Check sheet for the modelled part. Datum: model origin and axes. Units: mm. A direction names the side the tool comes from. Round coordinates to 2 decimals unless told otherwise and drop trailing zeros. Write each loop counter-clockwise with the first axis right and the second up, starting at its lowest first coordinate (ties: lowest second). Pieces come first, ordered by that corner, then holes. Notation, with made-up numbers: (-37, 14.5) -> (2, 14.5) arc R23 ccw to (2, 31.5) -> close; hole circle Ø6 at (-33.75, 49). An arc over 180 degrees is marked (long way). Use one line per item in the form item = value. Start each with the question number.
```python
from build123d import *

# Parameters (mm, degrees)
F0_W     = 60
F0_H     = 20
F2_R     = 5
F3_DEPTH = 20
F4_R     = 5


with BuildPart() as f1:
    # F0 (on Front) → F1 (revolve)
    with BuildSketch(Plane.XZ):
        with Locations((-30, 10)):
            Rectangle(F0_W, F0_H)
    revolve(axis=Axis((-30, 0, 0), (-1, 0, 0)))

    # F2
    f2_edges = [f1.edges().sort_by_distance(p)[0] for p in [
        (-60, 0, -20),
        (0, 0, -20),
    ]]
    fillet(f2_edges, radius=F2_R)

    # F3 (add): a face of the model
    f3_faces = [f1.faces().sort_by_distance(p)[0] for p in [
        (-60, 0, 0),
    ]]
    extrude(f3_faces, amount=F3_DEPTH)

    # F4
    f4_edges = [f1.edges().sort_by_distance(p)[0] for p in [
        (-60, 0, -15),
        (-80, 0, -15),
    ]]
    fillet(f4_edges, radius=F4_R)


solid = f1.part
```
1. Scan lines: probe 1 along X at (y, z) = (-6.5, -11.5); probe 2 along Y at (x, z) = (-34.5, -17.5); probe 3 along Z at (x, y) = (-60, 0). Record each from-to range of solid material in increasing order.
2. Tool access check on faces 1 (the face through (-80, 0, 0)), 2 (the face through (-69.251, 4.506, 14.307)). Record the directions out of +Z, -Z, +X, -X, +Y, -Y that give a thin tool (end or side, any length) a straight path to the whole face; none if there is none.
3. Sectioned sample at B-B (x = -51.5). Enter the section's corners in (y, z), and give its area (3 significant figures).
4. Depth check by flat-ended pin: pin 1 (10 mm diameter, centred on y = 14.5, z = -10.5, fed in from -X); pin 2 (4 mm diameter, centred on x = -60.5, z = 15, fed in from -Y); pin 3 (6 mm diameter, centred on y = -9.5, z = 5, fed in from +X); pin 4 (10 mm diameter, centred on x = -23.5, y = -12, fed in from +Z) (3 decimals). Enter the tip coordinate at first touch or a pass-through.
5. Sectioned sample at A-A (x = -68). Enter the section's corners in (y, z).
Returned:
q1.probe_1 = -78.83 to 0
q1.probe_2 = -9.68 to 9.68
q1.probe_3 = -16.59 to 16.59
q2.face_1 = +Z, -Z, -X, +Y, -Y
q2.face_2 = -X
q3.outline = circle Ø40 at (0, 0)
q3.area = 1,260 mm^2
q4.pin_1 = -79.07
q4.pin_2 = -11.77
q4.pin_3 = 0
q4.pin_4 = 18.735
q5.outline = circle Ø30 at (0, 0)
